Work out the finished part from the listing and answer in its coordinate system (mm). Face numbers are marked on the shaded views. A direction names the side the tool comes from. Round coordinates to 2 decimals unless told otherwise and drop trailing zeros. Write each loop counter-clockwise with the first axis right and the second up, starting at its lowest first coordinate (ties: lowest second). Pieces come first, ordered by that corner, then holes. Notation, with made-up numbers: M -1,-27 L 3,-27 A26 ccw 3,-13 Z; hole C -33.75,55 d2. An arc over 180 degrees is marked long. Answer in a Markdown table with one row per item.
```python
from build123d import *

# Parameters (mm, degrees)
SKETCH3_R            = 12.9
BOSS_EXTRUDE3_DEPTH  = 24
SKETCH5_W            = 8
SKETCH5_H            = 24
BOSS_EXTRUDE4_DEPTH  = 6
SKETCH7_R            = 2.4
BOSS_EXTRUDE5_DEPTH  = 28.8
SKETCH6_R            = 11.3
CUT_EXTRUDE1_DEPTH   = 6
REFERENCEW_W         = 23.783187338
REFERENCEW_H         = 9.6
REFERENCEW_W_2       = 25.0926284
REFERENCEW_H_2       = 9.9
CUT_EXTRUDE2_DEPTH   = 8
SKETCH8_R            = 2.4
BOSS_EXTRUDE6_DEPTH  = 1.6
LPATTERN1_COUNT      = 3
LPATTERN1_PITCH      = 8
LPATTERN1_COUNT_DIR2 = 2
LPATTERN1_PITCH_DIR2 = 8
SKETCH9_W            = 20.583187338
SKETCH9_H            = 12.8
CUT_EXTRUDE3_DEPTH   = 1.6
SHELL1_START         = -14.6
SHELL1_OUTLINE_W     = 4.8
SHELL1_OUTLINE_H     = 6.8
SHELL1_DEPTH         = 17.6
SHELL1_2_OUTLINE_W   = 4.8
SHELL1_2_OUTLINE_H   = 6
SHELL1_2_DEPTH       = 1.7
SHELL1_START_2       = -1.8
SHELL1_3_OUTLINE_R   = 0.8
SHELL1_3_DEPTH       = 4.8
SHELL1_START_3       = 3
SHELL1_4_OUTLINE_R   = 0.8
SHELL1_4_DEPTH       = 9.6
SHELL1_START_4       = -16.4
SHELL1_5_DEPTH       = 6.8
SHELL1_START_5       = 9.6
SHELL1_6_DEPTH       = 6.8
SHELL1_START_6       = -9.6
SHELL1_7_DEPTH       = 19.2
SHELL1_8_DEPTH       = 1.6
SHELL1_START_7       = 8
SHELL1_9_DEPTH       = 1.6
SHELL1_START_8       = -22.4
SHELL1_10_DEPTH      = 6
SHELL1_START_9       = 16.4
SHELL1_11_DEPTH      = 6


with BuildPart() as part:
    # Sketch3 → Boss-Extrude3 (new body)
    with BuildSketch(Plane.XY):
        Circle(SKETCH3_R)
    boss_extrude3 = extrude(amount=BOSS_EXTRUDE3_DEPTH)

    # Sketch5 → Boss-Extrude4 (add)
    with BuildSketch(Plane(origin=(0, -14.6, 0), x_dir=(1, 0, 0), z_dir=(0, 1, 0))):
        with Locations((0, -12)):
            Rectangle(SKETCH5_W, SKETCH5_H)
    boss_extrude4 = extrude(amount=BOSS_EXTRUDE4_DEPTH)

    # Sketch7 → Boss-Extrude5 (add)
    with BuildSketch(Plane.XZ.offset(14.6)):
        with Locations(Location((0, 12, 0), (0, 0, 270))):
            Circle(SKETCH7_R)
    boss_extrude5 = extrude(amount=-BOSS_EXTRUDE5_DEPTH)

    # Sketch6 → Cut-Extrude1 (cut)
    with BuildSketch(Plane.XY.offset(24)):
        Circle(SKETCH6_R)
    cut_extrude1 = extrude(amount=-CUT_EXTRUDE1_DEPTH, mode=Mode.SUBTRACT)

    # referencew → Cut-Extrude2 (cut)
    with BuildSketch(Plane(origin=(0, 0, 0), x_dir=(-1, 0, 0), z_dir=(0, 0, -1))):
        with Locations((0, -9.8)):
            Rectangle(REFERENCEW_W, REFERENCEW_H)
        with Locations((0, 7.95)):
            Rectangle(REFERENCEW_W_2, REFERENCEW_H_2)
    cut_extrude2 = extrude(amount=-CUT_EXTRUDE2_DEPTH, mode=Mode.SUBTRACT)

    # Mirror1: Boss-Extrude3, Boss-Extrude4, Boss-Extrude5, Cut-Extrude1, Cut-Extrude2 across Front Plane
    add(boss_extrude3.mirror(Plane.XY))
    add(boss_extrude4.mirror(Plane.XY))
    add(boss_extrude5.mirror(Plane.XY))
    add(cut_extrude1.mirror(Plane.XY), mode=Mode.SUBTRACT)
    add(cut_extrude2.mirror(Plane.XY), mode=Mode.SUBTRACT)

    # Sketch8 → Boss-Extrude6 (add)
    with BuildSketch(Plane(origin=(0, 3, 0), x_dir=(1, 0, 0), z_dir=(0, 1, 0))):
        with Locations(Location((8.5463142, 4, 0), (0, 0, 90))):
            Circle(SKETCH8_R)
    boss_extrude6 = extrude(amount=BOSS_EXTRUDE6_DEPTH)

    # LPattern1: Boss-Extrude6 3 × 2
    with Locations(*[(-i * LPATTERN1_PITCH, 0, j * LPATTERN1_PITCH_DIR2) for i in range(LPATTERN1_COUNT) for j in range(LPATTERN1_COUNT_DIR2) if (i, j) != (0, 0)]):
        add(boss_extrude6)

    # Sketch9 → Cut-Extrude3 (cut)
    with BuildSketch(Plane.XZ.offset(5)):
        Rectangle(SKETCH9_W, SKETCH9_H)
    extrude(amount=-CUT_EXTRUDE3_DEPTH, mode=Mode.SUBTRACT)

    # Shell1: read off the stored shape, not the designer's step
    # Shell1 outline → Shell1 (cut)
    with BuildSketch(Plane(origin=(0, 0, 0), x_dir=(1, 0, 0), z_dir=(0, 1, 0)).offset(SHELL1_START)):
        with Locations((0, 13)):
            Rectangle(SHELL1_OUTLINE_W, SHELL1_OUTLINE_H)
        with Locations((0, -13)):
            Rectangle(SHELL1_OUTLINE_W, SHELL1_OUTLINE_H)
    extrude(amount=SHELL1_DEPTH, mode=Mode.SUBTRACT)

    # Shell1 2 outline → Shell1 2 (cut)
    with BuildSketch(Plane(origin=(0, 0, 0), x_dir=(1, 0, 0), z_dir=(0, 1, 0)).offset(SHELL1_START)):
        with Locations((0, 19.4)):
            Rectangle(SHELL1_2_OUTLINE_W, SHELL1_2_OUTLINE_H)
        with Locations((0, -19.4)):
            Rectangle(SHELL1_2_OUTLINE_W, SHELL1_2_OUTLINE_H)
    extrude(amount=SHELL1_2_DEPTH, mode=Mode.SUBTRACT)

    # Shell1 3 outline → Shell1 3 (cut)
    with BuildSketch(Plane(origin=(0, 0, 0), x_dir=(1, 0, 0), z_dir=(0, 1, 0)).offset(SHELL1_START_2)):
        with Locations((8.5463142, 4)):
            Circle(SHELL1_3_OUTLINE_R)
        with Locations((8.5463142, -4)):
            Circle(SHELL1_3_OUTLINE_R)
        with Locations((0.5463142, 4)):
            Circle(SHELL1_3_OUTLINE_R)
        with Locations((0.5463142, -4)):
            Circle(SHELL1_3_OUTLINE_R)
        with Locations((-7.4536858, 4)):
            Circle(SHELL1_3_OUTLINE_R)
        with Locations((-7.4536858, -4)):
            Circle(SHELL1_3_OUTLINE_R)
    extrude(amount=SHELL1_3_DEPTH, mode=Mode.SUBTRACT)

    # Shell1 4 outline → Shell1 4 (cut)
    with BuildSketch(Plane(origin=(0, 0, 0), x_dir=(1, 0, 0), z_dir=(0, 1, 0)).offset(SHELL1_START_3)):
        with Locations((0, -12)):
            Circle(SHELL1_4_OUTLINE_R)
        with Locations((0, 12)):
            Circle(SHELL1_4_OUTLINE_R)
    extrude(amount=SHELL1_4_DEPTH, mode=Mode.SUBTRACT)

    # Shell1 5 outline → Shell1 5 (cut)
    with BuildSketch(Plane.XY.offset(SHELL1_START_4)):
        with BuildLine():
            Line((-2.4, -11.042191811), (-2.4, 3))
            Line((-2.4, 3), (2.4, 3))
            Line((2.4, 3), (2.4, -11.042191811))
            ThreePointArc((2.4, -11.042191811), (0, 11.3), (-2.4, -11.042191811))
        make_face()
    extrude(amount=SHELL1_5_DEPTH, mode=Mode.SUBTRACT)

    # Shell1 6 outline → Shell1 6 (cut)
    with BuildSketch(Plane.XY.offset(SHELL1_START_5)):
        with BuildLine():
            Line((-2.4, -11.042191811), (-2.4, 3))
            Line((-2.4, 3), (2.4, 3))
            Line((2.4, 3), (2.4, -11.042191811))
            ThreePointArc((2.4, -11.042191811), (0, 11.3), (-2.4, -11.042191811))
        make_face()
    extrude(amount=SHELL1_6_DEPTH, mode=Mode.SUBTRACT)

    # Shell1 7 outline → Shell1 7 (cut)
    with BuildSketch(Plane.XY.offset(SHELL1_START_6)):
        with BuildLine():
            ThreePointArc((-11.212938954, 1.4), (-11.298193722, -0.202036175), (-11.155716023, -1.8))
            Line((-11.155716023, -1.8), (11.155716023, -1.8))
            ThreePointArc((11.155716023, -1.8), (11.298193722, -0.202036175), (11.212938954, 1.4))
            Line((11.212938954, 1.4), (-11.212938954, 1.4))
        make_face()
    extrude(amount=SHELL1_7_DEPTH, mode=Mode.SUBTRACT)

    # Shell1 8 outline → Shell1 8 (cut)
    with BuildSketch(Plane.XY.offset(SHELL1_START_6)):
        with BuildLine():
            ThreePointArc((-11.155716023, -1.8), (-10.9951818, -2.606909506), (-10.776363023, -3.4))
            Line((-10.776363023, -3.4), (10.776363023, -3.4))
            ThreePointArc((10.776363023, -3.4), (10.9951818, -2.606909506), (11.155716023, -1.8))
            Line((11.155716023, -1.8), (-11.155716023, -1.8))
        make_face()
    extrude(amount=SHELL1_8_DEPTH, mode=Mode.SUBTRACT)

    # Shell1 9 outline → Shell1 9 (cut)
    with BuildSketch(Plane.XY.offset(SHELL1_START_7)):
        with BuildLine():
            ThreePointArc((-11.155716023, -1.8), (-10.9951818, -2.606909506), (-10.776363023, -3.4))
            Line((-10.776363023, -3.4), (10.776363023, -3.4))
            ThreePointArc((10.776363023, -3.4), (10.9951818, -2.606909506), (11.155716023, -1.8))
            Line((11.155716023, -1.8), (-11.155716023, -1.8))
        make_face()
    extrude(amount=SHELL1_9_DEPTH, mode=Mode.SUBTRACT)

    # Shell1 10 outline → Shell1 10 (cut)
    with BuildSketch(Plane.XY.offset(SHELL1_START_8)):
        with BuildLine():
            ThreePointArc((0, -12.9), (-1.205272262, -12.843571107), (-2.4, -12.674778105))
            Line((-2.4, -12.674778105), (-2.4, -12.9))
            Line((-2.4, -12.9), (0, -12.9))
        make_face()
        with BuildLine():
            ThreePointArc((2.4, -12.674778105), (1.205272262, -12.843571107), (0, -12.9))
            Line((0, -12.9), (2.4, -12.9))
            Line((2.4, -12.9), (2.4, -12.674778105))
        make_face()
    extrude(amount=SHELL1_10_DEPTH, mode=Mode.SUBTRACT)

    # Shell1 11 outline → Shell1 11 (cut)
    with BuildSketch(Plane.XY.offset(SHELL1_START_9)):
        with BuildLine():
            ThreePointArc((0, -12.9), (-1.205272262, -12.843571107), (-2.4, -12.674778105))
            Line((-2.4, -12.674778105), (-2.4, -12.9))
            Line((-2.4, -12.9), (0, -12.9))
        make_face()
        with BuildLine():
            ThreePointArc((2.4, -12.674778105), (1.205272262, -12.843571107), (0, -12.9))
            Line((0, -12.9), (2.4, -12.9))
            Line((2.4, -12.9), (2.4, -12.674778105))
        make_face()
    extrude(amount=SHELL1_11_DEPTH, mode=Mode.SUBTRACT)


solid = part.part
```
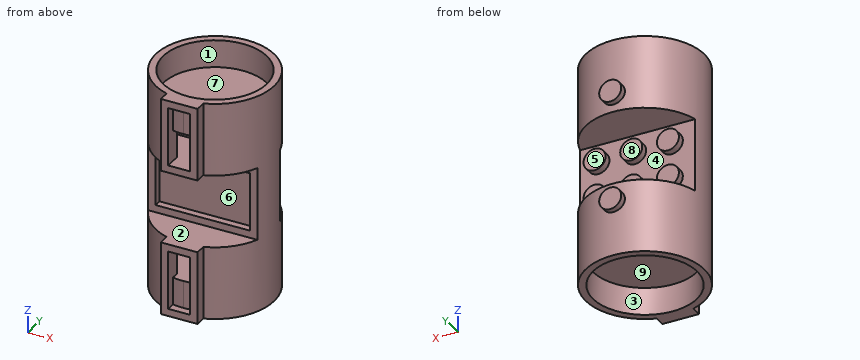
1. A tool of negligible diameter and unlimited length cuts with its end or side. For the marked faces 1, 2, 3, 4 and 5, from which of +Z, -Z, +X, -X, +Y, -Y can it reach the whole face along a straight path? Write none if from no direction.
Calculated:
| item | result |
|---|---|
| face 1 | +Z |
| face 2 | +X, -X, -Y |
| face 3 | -Z |
| face 4 | +Y |
| face 5 | +X, -X, +Y |
2. Determine the mould class of the marked faces 6, 7, 8 and 9 for opening direction Z: released by +Z, released by -Z, zero draft, split by the parting line, or undercut.
Calculated:
| item | result |
|---|---|
| face 6 | undercut |
| face 7 | released by +Z |
| face 8 | undercut |
| face 9 | released by -Z |
3. The part is cut by section D-D (z = 12). Determine the outline of the cut face in (x, y), plus the area to 3 significant figures.
Calculated:
| item | result |
|---|---|
| outline | M -4,-14.6 L -2.4,-14.6 L -2.4,-11.04 A11.3 cw -0.8,11.27 L -0.8,12.6 L 0.8,12.6 L 0.8,11.27 A11.3 cw 2.4,-11.04 L 2.4,-14.6 L 4,-14.6 L 4,-12.26 A12.9 ccw 2.4,12.67 L 2.4,14.2 L -2.4,14.2 L -2.4,12.67 A12.9 ccw -4,-12.26 Z |
| area | 125 mm² |
4. The part is cut by section C-C (y = 0). Determine the outline of the cut face in (x, z).
Calculated:
| item | result |
|---|---|
| outline | M -12.9,-24 L -11.3,-24 L -11.3,-18 L 11.3,-18 L 11.3,-24 L 12.9,-24 L 12.9,24 L 11.3,24 L 11.3,18 L -11.3,18 L -11.3,24 L -12.9,24 Z; hole M -11.3,-16.4 L 11.3,-16.4 L 11.3,16.4 L -11.3,16.4 Z |
5. Consider line 1 along Z through (x, y) = (-0.5, 5.75); line 2 along Z through (x, y) = (-7.5, 8.5); line 3 along Y through (x, z) = (10.5, 7.5). Determine where each line is inside the solid, lowest interval first. Write a range as from..to.
Calculated:
| item | result |
|---|---|
| line 1 | z = -18..-16.4, -9.6..-8, 8..9.6, 16.4..18 |
| line 2 | z = -24..-8, 8..24 |
| line 3 | y = -5..-1.8, 1.4..3 |
6. Given pin 1 (1 mm diameter, centred on y = 2, z = 7.5, fed in from -X); pin 2 (1.3 mm diameter, centred on x = 2.5, y = -2.5, fed in from -Z); pin 3 (11.5 mm diameter, centred on x = 3, y = -6, fed in from +Z); pin 4 (1.3 mm diameter, centred on x = -7.45, z = 4, fed in from -Y), each flat-ended and moving along its own axis, determine where each tip first touches the part or whether it passes through.
Calculated:
| item | result |
|---|---|
| pin 1 | stops at x = -12.81 |
| pin 2 | stops at z = -18 |
| pin 3 | stops at z = 24 |
| pin 4 | stops at y = -3.4 |
7. The part is cut by section A-A (y = -7). Determine the outline of the cut face in (x, z).
Calculated:
| item | result |
|---|---|
| outline | M -10.84,-24 L -8.87,-24 L -8.87,-18 L 8.87,-18 L 8.87,-24 L 10.84,-24 L 10.84,-8 L -10.84,-8 Z; M -10.84,8 L 10.84,8 L 10.84,24 L 8.87,24 L 8.87,18 L -8.87,18 L -8.87,24 L -10.84,24 Z; hole M -8.87,-16.4 L 8.87,-16.4 L 8.87,-9.6 L -8.87,-9.6 Z; hole M -8.87,9.6 L 8.87,9.6 L 8.87,16.4 L -8.87,16.4 Z |
8. The part is cut by section B-B (z = -20.5). Determine the outline of the cut face in (x, y).
Calculated:
| item | result |
|---|---|
| outline | M -4,-14.6 L -2.4,-14.6 L -2.4,-12.67 A12.9 ccw 2.4,-12.67 L 2.4,-14.6 L 4,-14.6 L 4,-12.26 A12.9 ccw long -4,-12.26 Z; hole C 0,0 d22.6 |
